Input: part model. Units: mm. Frame: model coordinates. A direction names the side the tool comes from. Coordinates: 2 decimals unless noted, no trailing zeros. Order: outer loops, then holes, each group sorted by start corner. A loop starts at its lowest first (then second) coordinate and runs counter-clockwise, first axis right, second up. Notation, with made-up numbers: (-16, 8) -> (17, 8) arc R13 cw to (17, 33) -> close; hole circle Ø8 at (61.5, 39). An arc over 180 degrees is marked (long way). Use one line per item in the form item = value. Start each with the question number.
1) Ray query, line 1 along X through (y, z) = (36, -43) (3 decimals); line 2 along X through (y, z) = (29, -14) (3 decimals); line 3 along Y through (x, z) = (212, -33) (1 decimal). Return the intervals inside material, ascending.
2) Draft query along Z for faces 6 (the flat face through (112, 35, 32.129)), 7 (the cylindrical face through (12.831, 31.011, -17.592)), 8 (the flat face through (34, -1.788, -23)). Return one class per face: pulls with the +Z half, pulls with the -Z half, needs draft (parallel to the pull), parting line crosses it, or undercut.
3) Section query B-B on y = 41. Count the separate pieces of the cut face and the enclosed holes in it, then the cut area to 3 significant figures.
4) Pin query (flat end, axial travel): pin 1 (10 mm diameter, centred on y = 17.5, z = -55.5, fed in from -X) (3 decimals); pin 2 (4 mm diameter, centred on x = 12.7, z = -59.91, fed in from -Y) (3 decimals); pin 3 (1 mm diameter, centred on x = 183, y = 4, fed in from -Z). Return the tip coordinate at first contact, or that it passes through.
5) Section query A-A on z = -66.5. Output: boundary loops of the cut face in (x, y) (3 decimals), then the cut area to 3 significant figures.
6) Section query C-C on x = 176. Output: boundary loops of the cut face in (y, z), then the cut area to 3 significant figures.
7) Access query for faces 1 (the cylindrical face through (208.12, 40.03, -78.773)), 2 (the flat face through (206, 47.425, -43)), 3 (the flat face through (22.025, 26, -52)), 4 (the cylindrical face through (110.5, 1.41, -10.7)), 5 (the flat face through (218.875, 25, -52)). Directions: +Z, -Z, +X, -X, +Y, -Y. A direction counts if a zero-diameter tool reaches every point of the face in a straight line with its end or side. Return the directions, or none.
from build123d import *

# Parameters (mm, degrees)
BOSS_EXTRUDE1_DEPTH = 222.25
BOSS_EXTRUDE3_DEPTH = 85
SKETCH15_R          = 2.349500000000014
CUT_EXTRUDE6_DEPTH  = 15
SKETCH16_R          = 5.499999999999996
SKETCH16_R_2        = 5.499999999999989
CUT_EXTRUDE7_DEPTH  = 224.37343312265227
BOSS_EXTRUDE5_DEPTH = 222.25
CUT_EXTRUDE3_DEPTH  = 222.25
BOSS_EXTRUDE6_DEPTH = 222.25
CUT_EXTRUDE4_REACH  = 245.691
SKETCH10_W          = 86.747166
SKETCH10_H          = 3.084529946162071
CHAMFER1_SIZE       = 3.5
CUT_EXTRUDE5_REACH  = 245.691
FILLET1_R           = 4
FILLET2_R           = 20
FILLET3_R           = 4


with BuildPart() as part:
    # Sketch1 → Boss-Extrude1 (new body)
    with BuildSketch(Plane(origin=(0, 0, 0), x_dir=(0, 0, -1), z_dir=(1, 0, 0))):
        Polygon((0, 0), (0, 50.8), (29.32939367483333, 0), align=None)
    extrude(amount=BOSS_EXTRUDE1_DEPTH)

    # Sketch3 → Boss-Extrude3 (add)
    with BuildSketch(Plane.XY):
        Polygon((218.875, 47.425), (200.22500000000002, 47.425), (200.22500000000002, 3.374999999999998), (218.875, 3.375), align=None)
    boss_extrude3 = extrude(amount=-BOSS_EXTRUDE3_DEPTH)

    # Sketch15 → Cut-Extrude6 (cut)
    with BuildSketch(Plane(origin=(0, 47.425, 0), x_dir=(1, 0, 0), z_dir=(0, 1, 0))):
        with Locations(Location((209.55000000000064, 59.90863352220276, 0), (0, 0, 270))):
            Circle(SKETCH15_R)
        with Locations(Location((209.55000000000064, 42.90863352220276, 0), (0, 0, 270))):
            Circle(SKETCH15_R)
        with Locations(Location((209.55000000000064, 76.90863352220276, 0), (0, 0, 270))):
            Circle(SKETCH15_R)
    cut_extrude6 = extrude(amount=-CUT_EXTRUDE6_DEPTH, mode=Mode.SUBTRACT)

    # Sketch16 → Cut-Extrude7 (cut, through all)
    with BuildSketch(Plane.ZY.offset(-200.22500000000002)):
        with Locations((-22.67268904895815, 33.11725062299641)):
            Circle(SKETCH16_R)
        with Locations((-32.67268904895816, 15.796742547307629)):
            Circle(SKETCH16_R_2)
    cut_extrude7 = extrude(amount=-CUT_EXTRUDE7_DEPTH, mode=Mode.SUBTRACT)

    # Mirror1: Boss-Extrude3, Cut-Extrude6, Cut-Extrude7 across plane
    add(boss_extrude3.mirror(Plane.ZY.offset(-111.125)))
    add(cut_extrude6.mirror(Plane.ZY.offset(-111.125)), mode=Mode.SUBTRACT)
    add(cut_extrude7.mirror(Plane.ZY.offset(-111.125)), mode=Mode.SUBTRACT)

    # Sketch7 → Boss-Extrude5 (add)
    with BuildSketch(Plane(origin=(222.25, 0, 0), x_dir=(0, 0, -1), z_dir=(1, 0, 0))):
        Polygon((0, 50.8), (-32.128627, 50.79999999999999), (-32.128626999999994, 22.043620610825506), (9.32939367483333, 0), (29.32939367483333, 0), align=None)
    extrude(amount=-BOSS_EXTRUDE5_DEPTH)

    # Sketch8 → Cut-Extrude3 (cut)
    with BuildSketch(Plane(origin=(222.25, 0, 0), x_dir=(0, 0, -1), z_dir=(1, 0, 0))):
        Polygon((0, 4.960526608591835), (9.32939367483333, 0), (0, 0), align=None)
    extrude(amount=-CUT_EXTRUDE3_DEPTH, mode=Mode.SUBTRACT)

    # Sketch9 → Boss-Extrude6 (add)
    with BuildSketch(Plane(origin=(222.25, 0, 0), x_dir=(0, 0, -1), z_dir=(1, 0, 0))):
        Polygon((32.52939367483333, -1.7875), (12.691192231639896, -1.7875000000000023), (9.32939367483333, 0), (29.32939367483333, 0), (29.44486372867126, -0.2000000000000005), (32.52939367483333, -0.2), align=None)
    extrude(amount=-BOSS_EXTRUDE6_DEPTH)

    # Sketch10 → Cut-Extrude4 (cut, up to next)
    with BuildSketch(Plane.XZ.offset(1.7875000000000039), mode=Mode.PRIVATE) as cut_extrude4_sk1:
        Polygon((218.872166, -32.52939367483333), (222.25, -28.82939367483333), (222.25, -32.52939367483333), align=None)
    cut_extrude4_tool1 = extrude(cut_extrude4_sk1.sketch, amount=-CUT_EXTRUDE4_REACH, mode=Mode.PRIVATE) & part.part
    # Sketch10 → Cut-Extrude4 (cut, up to next)
    with BuildSketch(Plane.XZ.offset(1.7875000000000039), mode=Mode.PRIVATE) as cut_extrude4_sk2:
        with Locations((154.49858300000002, -30.987128701752294)):
            Rectangle(SKETCH10_W, SKETCH10_H)
    cut_extrude4_tool2 = extrude(cut_extrude4_sk2.sketch, amount=-CUT_EXTRUDE4_REACH, mode=Mode.PRIVATE) & part.part
    cut_extrude4_1 = cut_extrude4_tool1.solids().sort_by_distance((221.124055, -1.7875, -31.29606))[0]
    add(cut_extrude4_1, mode=Mode.SUBTRACT)
    cut_extrude4_2 = cut_extrude4_tool2.solids().sort_by_distance((154.498583, -1.7875, -30.987129))[0]
    add(cut_extrude4_2, mode=Mode.SUBTRACT)
    cut_extrude4 = cut_extrude4_1 + cut_extrude4_2  # Cut-Extrude4 as one shape, for the pattern or mirror that repeats it

    # Mirror2: Cut-Extrude4 across plane
    add(cut_extrude4.mirror(Plane.ZY.offset(-111.125)), mode=Mode.SUBTRACT)

    # Chamfer1
    # the kernel refuses this chamfer: 3.5 mm, written as the material it takes off along each edge
    with BuildSketch(Plane(origin=(24.37783399999998, -10.788390457880682, -32.52939367483333), x_dir=(-0.9996219169112968, 0, -0.027495876610586126), z_dir=(0, 1, 1.7e-16))) as chamfer1_piece_1_section:
        Polygon((CHAMFER1_SIZE * 0.999621916911, CHAMFER1_SIZE * 0.0274958766106), (-CHAMFER1_SIZE * 0.0274958766106, CHAMFER1_SIZE * 0.999621916911), (0, 0), align=None)
    chamfer1_piece_1 = extrude(amount=10.588390457880683, mode=Mode.PRIVATE)
    chamfer1_piece_1 = split(chamfer1_piece_1, bisect_by=Plane(origin=(23.984976555626393, -1.314391432651377, -29.444863728671262), z_dir=(0, 1.7e-16, -1)), keep=Keep.TOP, mode=Mode.PRIVATE)
    add(chamfer1_piece_1, mode=Mode.SUBTRACT)
    with BuildSketch(Plane(origin=(197.87216600000002, -10.788390457880718, -32.52939367483333), x_dir=(-0.02749587661059007, 0, 0.9996219169112966), z_dir=(0, 1, 1.7e-16))) as chamfer1_piece_2_section:
        Polygon((CHAMFER1_SIZE * 0.999621916911, CHAMFER1_SIZE * 0.0274958766106), (-CHAMFER1_SIZE * 0.0274958766106, CHAMFER1_SIZE * 0.999621916911), (0, 0), align=None)
    chamfer1_piece_2 = extrude(amount=10.588390457880719, mode=Mode.PRIVATE)
    chamfer1_piece_2 = split(chamfer1_piece_2, bisect_by=Plane(origin=(198.26502344437364, -1.3143914326513721, -29.444863728671262), z_dir=(0, 1.7e-16, -1)), keep=Keep.TOP, mode=Mode.PRIVATE)
    add(chamfer1_piece_2, mode=Mode.SUBTRACT)

    # Cut-Extrude5: up to this plane
    cut_extrude5_end = Plane(origin=(222.25, 50.8, 0), z_dir=(0, -0.5000000000000044, 0.8660254037844362))
    # Sketch11 → Cut-Extrude5 (cut, up to the surface)
    with BuildSketch(Plane.XZ.offset(1.7875000000000039), mode=Mode.PRIVATE) as cut_extrude5_sk1:
        Polygon((66.12499999999999, -29.444863728671255), (156.125, -29.444863728671255), (156.125, -12.691192231639896), (66.12500000000001, -12.691192231639896), align=None)
    cut_extrude5_tool1 = split(extrude(cut_extrude5_sk1.sketch, amount=-CUT_EXTRUDE5_REACH, mode=Mode.PRIVATE), bisect_by=cut_extrude5_end, keep=Keep.BOTH, mode=Mode.PRIVATE)
    add(cut_extrude5_tool1.solids().sort_by_distance((111.125, -1.7875, -21.068028))[0], mode=Mode.SUBTRACT)

    # Fillet1
    fillet1_edges = [part.edges().sort_by_distance(p)[0] for p in [
        (111.125, -1.7875000000000016, -12.691192231639896),
    ]]
    fillet(fillet1_edges, radius=FILLET1_R)

    # Fillet2
    fillet2_edges = [part.edges().sort_by_distance(p)[0] for p in [
        (222.25, 36.42181030541275, 32.128627),
        (0, 36.42181030541275, 32.128627),
    ]]
    fillet(fillet2_edges, radius=FILLET2_R)

    # Fillet3
    fillet3_edges = [part.edges().sort_by_distance(p)[0] for p in [
        (222.25, 50.8, 6.064313500000003),
        (0, 50.8, 6.0643135000000035),
        (111.125, 50.79999999999999, 32.128627),
        (216.39213562373095, 50.8, 26.270762623730953),
        (5.857864376269047, 50.8, 26.27076262373096),
    ]]
    fillet(fillet3_edges, radius=FILLET3_R)


solid = part.part
Answers below:
q1.line_1 = 3.375 to 10.352, 15.048 to 22.025, 200.225 to 207.202, 211.898 to 218.875
q1.line_2 = 3.375 to 22.025, 200.225 to 218.875
q1.line_3 = 3.4 to 10.3, 21.3 to 47.4
q2.face_6 = pulls with the +Z half
q2.face_7 = undercut
q2.face_8 = needs draft
q3.separate_pieces = 1
q3.enclosed_holes = 6
q3.area = 11,100 mm^2
q4.pin_1 = 3.375
q4.pin_2 = 3.375
q4.pin_3 = -27.31
q5.outline = (3.375, 3.375) -> (22.025, 3.375) -> (22.025, 47.425) -> (3.375, 47.425) -> close; (200.225, 3.375) -> (218.875, 3.375) -> (218.875, 47.425) -> (200.225, 47.425) -> close
q5.area = 1,640 mm^2
q6.outline = (-1.79, -29.44) -> (-0.2, -29.44) -> (50.8, 0) -> (50.8, 28.13) arc R4 ccw to (46.8, 32.13) -> (22.04, 32.13) -> (-1.79, -12.69) -> close
q6.area = 1,950 mm^2
q7.face_1 = +Y
q7.face_2 = -Z, +X, -X, +Y
q7.face_3 = -Z, +Y
q7.face_4 = -Y
q7.face_5 = -Z, +X, +Y
